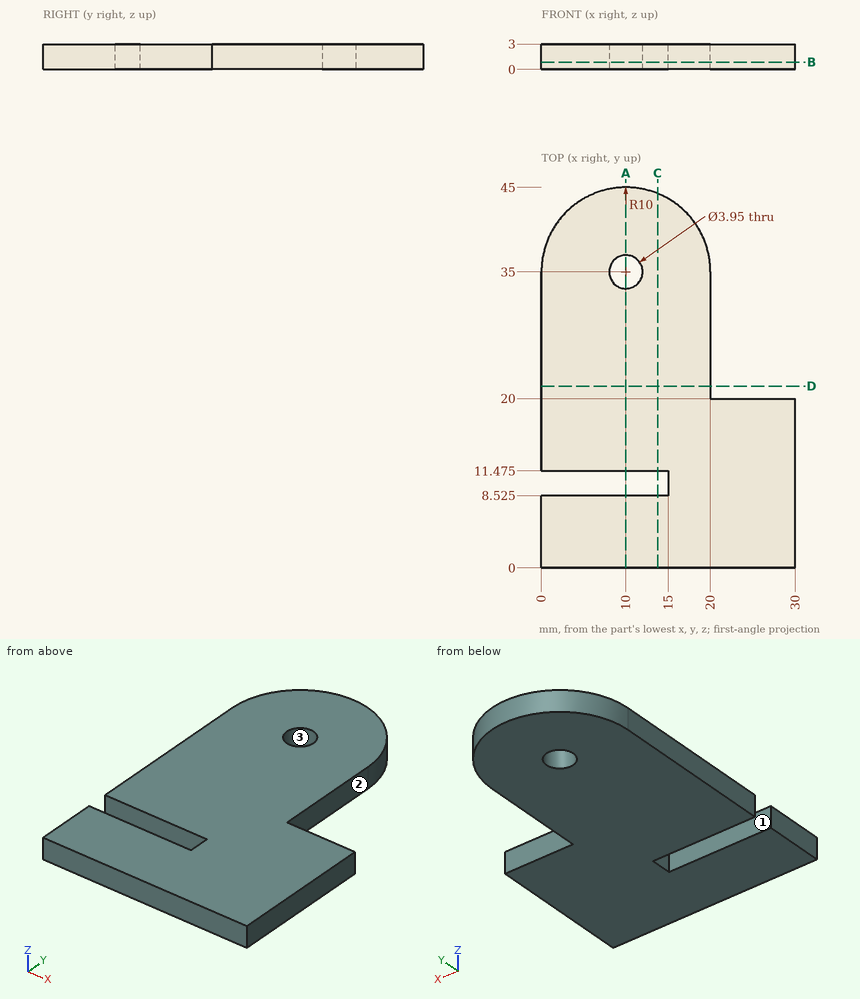
Could you check a few things on this drawing? It's one solid part, dimensions in mm from its lowest x, y, z. A direction names the side the tool comes from. Round coordinates to 2 decimals unless told otherwise and drop trailing zeros. Write each loop counter-clockwise with the first axis right and the second up, starting at its lowest first coordinate (ties: lowest second). Pieces come first, ordered by that corner, then holes. Notation, with made-up numbers: (55.25, 9) -> (114.25, 9) arc R32 ccw to (114.25, 42) -> close; hole circle Ø7 at (22, 56.25). An arc over 180 degrees is marked (long way). Use one line per item in the form item = value. Start each with the question number.
Q1. I'm going to push a flat-ended pin straight in: P1, Ø1.5, axis at x = 24, z = 1.5, coming from the +Y side. Where does the tip first touch, or does it pass through?
Q2. Imagine slicing it at A-A (x = 10). Please give me the cut outline in (y, z) (3 decimals).
Q3. Which directions (+Z, -Z, +X, -X, +Y, -Y) give clear straight access to the entire face, cutting with the end or side of a thin tool? Please do the marked faces 1, 2 and 3.
Q4. Imagine slicing it at B-B (z = 0.85). Please give me the cut outline in (x, y) (3 decimals), then the cut area to 3 significant figures.
Q5. Imagine slicing it at C-C (x = 13.75). Please give me the cut outline in (y, z) (3 decimals).
Q6. If I drill on probe 1 along Y at (x, z) = (10, 0.6) (3 decimals); probe 2 along Y at (x, z) = (11.25, 1.75) (3 decimals); probe 3 along X at (y, z) = (28, 1), over which ranges is the centre line in solid material (lowest first)? Write a range as [from, to].
Q7. Imagine slicing it at D-D (y = 21.5). Please give me the cut outline in (x, z), then the cut area to 3 significant figures.
Worked out:
q1.P1 = 20
q2.outline = (0, 0) -> (8.525, 0) -> (8.525, 3) -> (0, 3) -> close; (11.475, 0) -> (33.025, 0) -> (33.025, 3) -> (11.475, 3) -> close; (36.975, 0) -> (45, 0) -> (45, 3) -> (36.975, 3) -> close
q3.face_1 = +Z, -Z, -X
q3.face_2 = +Z, -Z, +X, +Y
q3.face_3 = +Z, -Z
q4.outline = (0, 0) -> (30, 0) -> (30, 20) -> (20, 20) -> (20, 35) arc R10 ccw to (0, 35) -> (0, 11.475) -> (15, 11.475) -> (15, 8.525) -> (0, 8.525) -> close; hole circle Ø3.95 at (10, 35)
q4.area = 1,000 mm^2
q5.outline = (0, 0) -> (8.525, 0) -> (8.525, 3) -> (0, 3) -> close; (11.475, 0) -> (44.27, 0) -> (44.27, 3) -> (11.475, 3) -> close
q6.probe_1 = [0, 8.525], [11.475, 33.025], [36.975, 45]
q6.probe_2 = [0, 8.525], [11.475, 33.471], [36.529, 44.922]
q6.probe_3 = [0, 20]
q7.outline = (0, 0) -> (20, 0) -> (20, 3) -> (0, 3) -> close
q7.area = 60.0 mm^2
